For this review, use the dimensioned drawing (mm, ordinates from the lowest corner) and the shaded views. A direction names the side the tool comes from. Give positions to 0.01 mm unless a question says otherwise; leave off trailing zeros. Loops run counter-clockwise (first coordinate to the right, second up) from the corner with the lowest first, then second, coordinate; pieces in that order, holes last. Notation, with made-up numbers: (71.25, -12.75) - (98.25, -12.75) arc R29 ccw to (98.25, 15.25) - close; hole circle Ø11 at (62.5, 65.5). An arc over 180 degrees is marked (long way). Write each question's results on one line, items separated by ' | '.
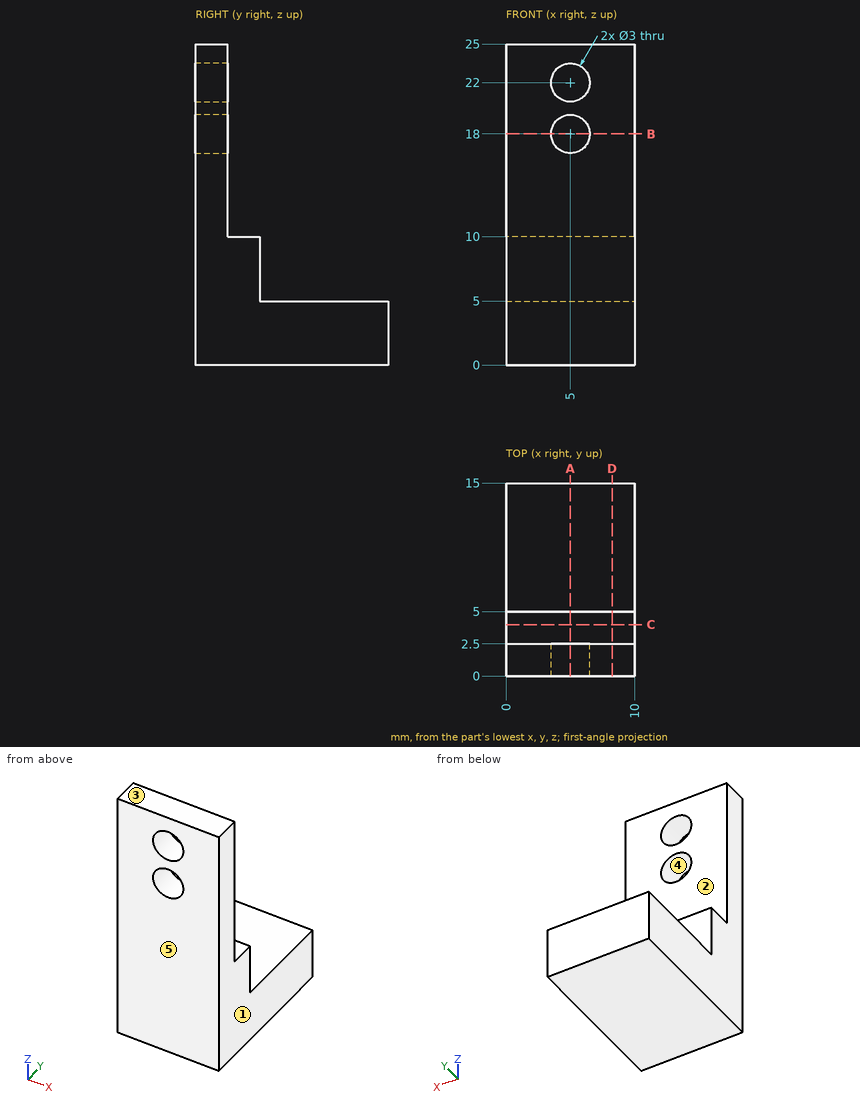
Item 1: Tool access review of the marked faces 1 and 2: name each direction out of +Z, -Z, +X, -X, +Y, -Y from which nothing blocks a thin tool from reaching the whole face with its end or side.
Output values:
face 1: +Z, -Z, +X, +Y, -Y | face 2: +Z, +X, -X, +Y
Item 2: Clearance check with flat-ended pins moving along their axes: P1, Ø5.5, axis at x = 5.5, z = 8.5, coming from the +Y side; P2, Ø1.5, axis at x = 6, z = 12.5, coming from the +Y side; P3, Ø3, axis at x = 6.5, y = 12, coming from the +Z side; P4, Ø3, axis at y = 5, z = 12, coming from the +X side. State where each tip first meets the part, or that it passes through.
Output values:
P1: stops at y = 5 | P2: stops at y = 2.5 | P3: stops at z = 5 | P4: passes through
Item 3: Draft analysis for pull direction Z (two halves, no side actions). For the marked faces 3, 4 and 5, state which applies: +Z half, -Z half, draft (parallel to the pull), parting line (faces both ways), or undercut.
Output values:
face 3: +Z half | face 4: undercut | face 5: draft
Item 4: We need section C-C on y = 4. Give the boundary of the cut face in (x, z).
Output values:
outline: (0, 0) - (10, 0) - (10, 10) - (0, 10) - close
Item 5: We need section A-A on x = 5. Give the boundary of the cut face in (y, z).
Output values:
outline: (0, 0) - (15, 0) - (15, 5) - (5, 5) - (5, 10) - (2.5, 10) - (2.5, 16.5) - (0, 16.5) - close; (0, 19.5) - (2.5, 19.5) - (2.5, 20.5) - (0, 20.5) - close; (0, 23.5) - (2.5, 23.5) - (2.5, 25) - (0, 25) - close
Item 6: Wall thickness on probe 1 along X at (y, z) = (0.9, 18); probe 2 along Y at (x, z) = (5, 12); probe 3 along Z at (x, y) = (6.5, 12.5): over which ranges is each line inside the solid? List them lowest first.
Output values:
probe 1: x = 0 to 3.5, 6.5 to 10 | probe 2: y = 0 to 2.5 | probe 3: z = 0 to 5
Item 7: We need section B-B on z = 18. Give the boundary of the cut face in (x, y).
Output values:
outline: (0, 0) - (3.5, 0) - (3.5, 2.5) - (0, 2.5) - close; (6.5, 0) - (10, 0) - (10, 2.5) - (6.5, 2.5) - close
Item 8: We need section D-D on x = 8.25. Give the boundary of the cut face in (y, z), then the cut area to 4 significant figures.
Output values:
outline: (0, 0) - (15, 0) - (15, 5) - (5, 5) - (5, 10) - (2.5, 10) - (2.5, 25) - (0, 25) - close | area: 137.5 mm²
